Answer from the drawing. Dimensions are ordinates in mm from the lowest x, y and z of the part. Give positions to 0.01 mm unless a question says otherwise; leave off trailing zeros. Order: outer loops, then holes, each group sorted by start corner. A loop starts at its lowest first (then second) coordinate and runs counter-clockwise, first axis right, second up.
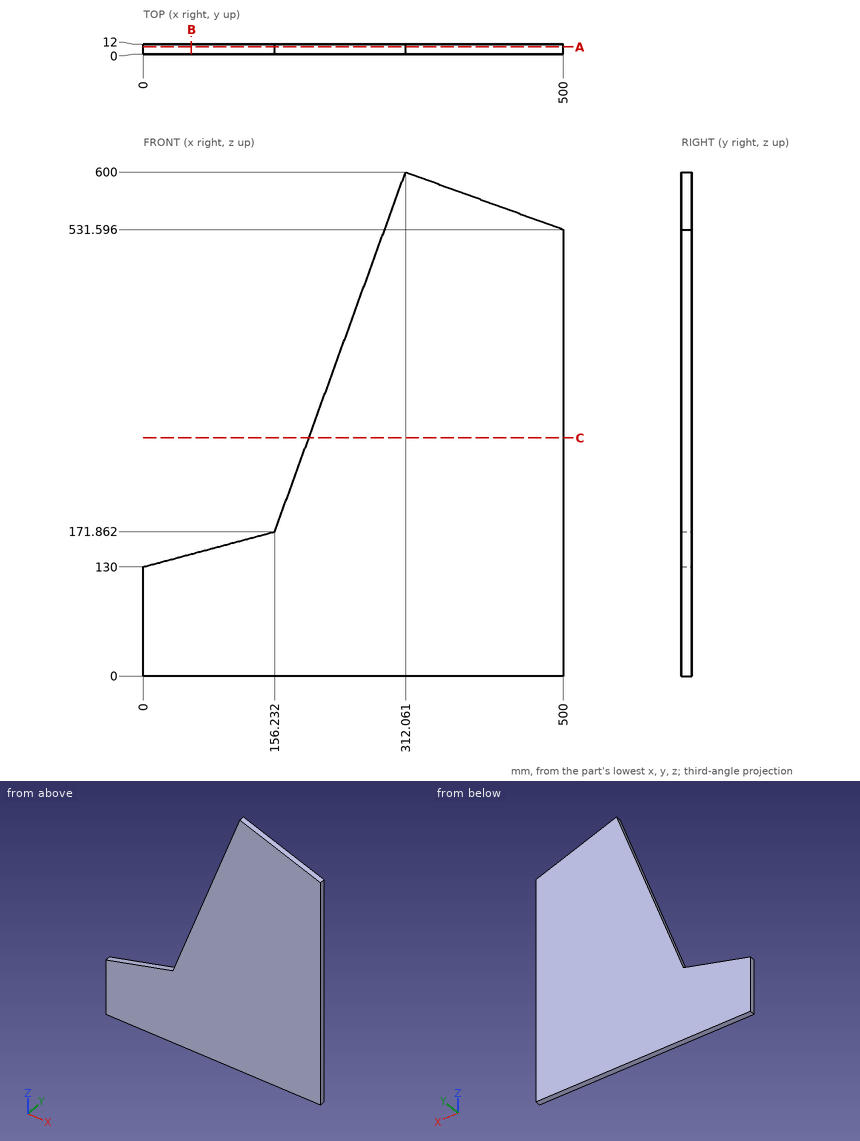
1) The part is cut by section C-C on z = 283.5. Determine the outline of the cut face in (x, y) (1 decimal).
Final values:
outline: (196.9, 0) - (500, 0) - (500, 12) - (196.9, 12) - close
2) Given pin 1 (1 mm diameter, centred on x = 133.5, y = 7, fed in from +Z) (1 decimal), flat-ended and moving along its own axis, determine where the tip first touches the part or whether it passes through.
Final values:
pin 1: stops at z = 165.9
3) The part is cut by section A-A on y = 8.5. Determine the outline of the cut face in (x, z).
Final values:
outline: (0, 0) - (500, 0) - (500, 531.6) - (312.06, 600) - (156.23, 171.86) - (0, 130) - close
4) The part is cut by section B-B on x = 57. Determine the outline of the cut face in (y, z).
Final values:
outline: (0, 0) - (12, 0) - (12, 145.27) - (0, 145.27) - close
5) Consider L1, parallel to X at y = 1, z = 296.5 (1 decimal); L2, parallel to X at y = 7, z = 275.5; L3, parallel to Z at x = 460, y = 2.5 (1 decimal). Determine where each line is inside the solid, lowest interval first.
Final values:
L1: x = 201.6 to 500
L2: x = 193.95 to 500
L3: z = 0 to 546.2
